from build123d import *

# Parameters (mm, degrees)
SKETCH1_W           = 300
SKETCH1_H           = 300
SKETCH1_W_2         = 228
SKETCH1_H_2         = 252
BOSS_EXTRUDE1_DEPTH = 8
CUT_EXTRUDE1_DEPTH  = 213.282830205
CUT_EXTRUDE2_START  = -15.3
SKETCH3_R           = 1.5
CUT_EXTRUDE2_DEPTH  = 15.3
MIRROR4_START       = -151
MIRROR4_OUTLINE_R   = 1.5
MIRROR4_DEPTH       = 284.7
MIRROR4_2_OUTLINE_R = 1.5
MIRROR4_2_DEPTH     = 17.3
MIRROR4_START_2     = -1
MIRROR4_3_DEPTH     = 10
SKETCH4_R           = 6
CUT_EXTRUDE3_DEPTH  = 213.282830205


with BuildPart() as part:
    # Sketch1 → Boss-Extrude1 (new body)
    with BuildSketch(Plane(origin=(0, 0, 0), x_dir=(1, 0, 0), z_dir=(0, 1, 0))):
        Rectangle(SKETCH1_W, SKETCH1_H)
        Rectangle(SKETCH1_W_2, SKETCH1_H_2, mode=Mode.SUBTRACT)
    extrude(amount=BOSS_EXTRUDE1_DEPTH)

    # Sketch2 → Cut-Extrude1 (cut, through all)
    with BuildSketch(Plane(origin=(0, 0, 0), x_dir=(1, 0, 0), z_dir=(0, 1, 0))):
        with BuildLine():
            Line((133.7, 150), (134.7, 150))
            Line((134.7, 150), (134.7, 139.959026766))
            ThreePointArc((134.7, 139.959026766), (133.799301132, 128.003357609), (133.7, 139.992495307))
            Line((133.7, 139.992495307), (133.7, 150))
        make_face()
    cut_extrude1 = extrude(amount=CUT_EXTRUDE1_DEPTH, mode=Mode.SUBTRACT)

    # Sketch3 → Cut-Extrude2 (cut)
    with BuildSketch(Plane(origin=(150, 0, 0), x_dir=(0, 0, -1), z_dir=(1, 0, 0)).offset(CUT_EXTRUDE2_START)):
        with Locations((146, 4)):
            Circle(SKETCH3_R)
    cut_extrude2 = extrude(amount=CUT_EXTRUDE2_DEPTH, mode=Mode.SUBTRACT)

    # Mirror3: Cut-Extrude1, Cut-Extrude2 across plane
    add(cut_extrude1.mirror(Plane.XY), mode=Mode.SUBTRACT)
    add(cut_extrude2.mirror(Plane.XY), mode=Mode.SUBTRACT)

    # Mirror4: read off the stored shape, not the designer's step
    # Mirror4 outline → Mirror4 (cut)
    with BuildSketch(Plane.YZ.offset(MIRROR4_START)):
        with Locations((4, -146)):
            Circle(MIRROR4_OUTLINE_R)
    extrude(amount=MIRROR4_DEPTH, mode=Mode.SUBTRACT)

    # Mirror4 2 outline → Mirror4 2 (cut)
    with BuildSketch(Plane.YZ.offset(MIRROR4_START)):
        with Locations((4, 146)):
            Circle(MIRROR4_2_OUTLINE_R)
    extrude(amount=MIRROR4_2_DEPTH, mode=Mode.SUBTRACT)

    # Mirror4 3 outline → Mirror4 3 (cut)
    with BuildSketch(Plane(origin=(0, 0, 0), x_dir=(1, 0, 0), z_dir=(0, 1, 0)).offset(MIRROR4_START_2)):
        with BuildLine():
            ThreePointArc((-134.7, 139.959026766), (-133.799301125, 128.003357609), (-133.7, 139.992495307))
            Line((-133.7, 139.992495307), (-133.7, 150))
            Line((-133.7, 150), (-134.7, 150))
            Line((-134.7, 150), (-134.7, 139.959026766))
        make_face()
        with BuildLine():
            Line((-133.7, -150), (-133.7, -139.992495307))
            ThreePointArc((-133.7, -139.992495307), (-133.799301125, -128.003357609), (-134.7, -139.959026766))
            Line((-134.7, -139.959026766), (-134.7, -150))
            Line((-134.7, -150), (-133.7, -150))
        make_face()
    extrude(amount=MIRROR4_3_DEPTH, mode=Mode.SUBTRACT)

    # Sketch4 → Cut-Extrude3 (cut, through all)
    with BuildSketch(Plane(origin=(0, 0, 0), x_dir=(1, 0, 0), z_dir=(0, 1, 0))):
        with Locations(Location((-128, 0, 0), (0, 0, 270))):
            Circle(SKETCH4_R)
    cut_extrude3 = extrude(amount=CUT_EXTRUDE3_DEPTH, mode=Mode.SUBTRACT)

    # Mirror5: Cut-Extrude3 across plane
    add(cut_extrude3.mirror(Plane(origin=(0, 0, 0), x_dir=(0, 0, 1), z_dir=(1, 0, 0))), mode=Mode.SUBTRACT)


solid = part.part
Model file for the job. Use its own axes, mm. A direction names the side the tool comes from. Round coordinates to 2 decimals unless told otherwise and drop trailing zeros. Loops run counter-clockwise (first coordinate to the right, second up) from the corner with the lowest first, then second, coordinate; pieces in that order, holes last. Notation, with made-up numbers: (26, 44.5) -> (42, 44.5) arc R23 ccw to (42, 82.5) -> close; hole circle Ø6 at (11.5, 12.25). An arc over 180 degrees is marked (long way). Answer as CSV lines item,"result". Start each with the question number.
1) Slice it at D-D (z = 0). List the corners of the cut face in (x, y), plus the area to 3 significant figures.
2) Slice it at B-B (z = -134). List the corners of the cut face in (x, y).
3) Slice it at C-C (y = 1.25). List the corners of the cut face in (x, z).
4) Mould opens along X. For faces 1 (the face through (-134, 4, 128)), 2 (the face through (150, 4, 2)), 3 (the face through (142, 4, -150)), 4 (the face through (-150, 4, 2)) say: +X half, -X half, draft (parallel to the pull), parting line (faces both ways), or undercut.
5) Tool access for faces 5 (the face through (-114, 4, 2)), 6 (the face through (-133.7, 4, -144)), 7 (the face through (-142, 4, -150)), 8 (the face through (-134.7, 4, 144)): list every direction of +Z, -Z, +X, -X, +Y, -Y with a clear straight run to the whole face (end or side of a thin tool).
6) Slice it at A-A (x = 46.5). List the corners of the cut face in (y, z).
7) Probe line 1 along X through (y, z) = (2.5, -134); line 2 along Z through (x, y) = (-112, 5.25); line 3 along Z through (x, y) = (16, 1.25). List the from-to ranges inside material, lowest first.
Filled in:
1,outline,"(-150, 0) -> (-134, 0) -> (-134, 8) -> (-150, 8) -> close; (-122, 0) -> (-114, 0) -> (-114, 8) -> (-122, 8) -> close; (114, 0) -> (122, 0) -> (122, 8) -> (114, 8) -> close; (134, 0) -> (150, 0) -> (150, 8) -> (134, 8) -> close"
1,area,"384 mm2"
2,outline,"(-150, 0) -> (-140, 0) -> (-140, 8) -> (-150, 8) -> close; (-128, 0) -> (128, 0) -> (128, 8) -> (-128, 8) -> close; (140, 0) -> (150, 0) -> (150, 8) -> (140, 8) -> close"
3,outline,"(-150, -150) -> (-134.7, -150) -> (-134.7, -139.96) arc R6 cw (long way) to (-133.7, -139.99) -> (-133.7, -150) -> (133.7, -150) -> (133.7, -139.99) arc R6 cw (long way) to (134.7, -139.96) -> (134.7, -150) -> (150, -150) -> (150, 150) -> (134.7, 150) -> (134.7, 139.96) arc R6 cw (long way) to (133.7, 139.99) -> (133.7, 150) -> (-133.7, 150) -> (-133.7, 139.99) arc R6 cw (long way) to (-134.7, 139.96) -> (-134.7, 150) -> (-150, 150) -> close; hole circle Ø12 at (-128, 0); hole (-114, -126) -> (114, -126) -> (114, 126) -> (-114, 126) -> close; hole circle Ø12 at (128, 0)"
4,face 1,"undercut"
4,face 2,"+X half"
4,face 3,"draft"
4,face 4,"-X half"
5,face 5,"+Y, -Y"
5,face 6,"-Z, +Y, -Y"
5,face 7,"-Z, +X, -X, +Y, -Y"
5,face 8,"+Z, +Y, -Y"
6,outline,"(0, -150) -> (8, -150) -> (8, -126) -> (0, -126) -> close; (0, 126) -> (8, 126) -> (8, 150) -> (0, 150) -> close; hole circle Ø3 at (4, -146)"
7,line 1,"x = -150 to -140, -128 to 128, 140 to 150"
7,line 2,"z = -150 to -146.83, -145.17 to -126, 126 to 150"
7,line 3,"z = -150 to -126, 126 to 150"
